Verification items for the finished model (mm, model axes). Coordinates: 2 decimals unless noted, no trailing zeros. Write each loop counter-clockwise with the first axis right and the second up, starting at its lowest first coordinate (ties: lowest second). Pieces come first, ordered by that corner, then holes. Notation, with made-up numbers: (70, -32.5) - (117, -32.5) arc R13 cw to (117, -17.5) - close; hole circle Ø3 at (-0.5, -23). An arc over 180 degrees is marked (long way). Answer as CSV lines item,"result". Start each with the question number.
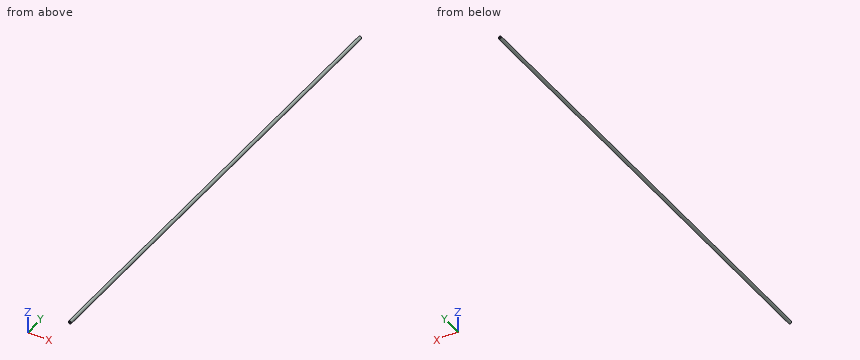
Autodesk Inventor part; units mm, degrees
ref_plane "YZ Plane" through (0, 0, 0) normal (1, 0, 0) x (0, 1, 0)
ref_plane "XZ Plane" through (0, 0, 0) normal (0, 1, 0) x (-1, 0, 0)
ref_plane "XY Plane" through (0, 0, 0) normal (0, 0, 1) x (1, 0, 0)
sketch "Sketch1" plane through (0, 0, 0) normal (0, 1, 0) x (-1, 0, 0)
  circle A0 centre (0, 0) radius 7
  circle A1 centre (0, 0) radius 3
  dimension "d0" = 14
  dimension "d1" = 6
extrude "Extrusion1" add sketch "Sketch1" along normal blind 1000 contours A0 | A1
extrude "Extrusion2" cut sketch "Sketch1" along normal blind 50 contours A1
chamfer "Chamfer1" distance 1 angle 45 1 edges at (7, 0, 0)
mirror "Mirror1" about plane through (0, 1000, 0) normal (0, 1, 0) of "Extrusion1", "Extrusion2", "Chamfer1"
properties part number "Tengely"
1. Cross-section at B-B (z = 0). Record the cut outline in (x, y), and give its area (3 significant figures).
2. Scan lines: line 1 along Z through (x, y) = (0, 38.5); line 2 along Z through (x, y) = (-1.75, 421); line 3 along X through (y, z) = (581, -1). Record each from-to range of solid material in increasing order. Write a range as from..to.
3. Depth check by flat-ended pin: P1, Ø5, axis at x = 0, z = 0, coming from the +Y side; P2, Ø1, axis at y = 1084.5, z = -4.5, coming from the -X side; P3, Ø3.5, axis at x = 0, z = 0, coming from the -Y side. Enter the tip coordinate at first touch or a pass-through.
4. Cross-section at C-C (y = 1081). Record the cut outline in (x, z).
5. Cross-section at A-A (x = 0). Record the cut outline in (y, z).
Completed:
1,outline,"(-7, 1) - (-6, 0) - (-3, 0) - (-3, 50) - (3, 50) - (3, 0) - (6, 0) - (7, 1) - (7, 1999) - (6, 2000) - (3, 2000) - (3, 1950) - (-3, 1950) - (-3, 2000) - (-6, 2000) - (-7, 1999) - close"
1,area,"27,400 mm2"
2,line 1,"z = -7..-3, 3..7"
2,line 2,"z = -6.78..6.78"
2,line 3,"x = -6.93..6.93"
3,P1,"stops at y = 1950"
3,P2,"stops at x = -5.74"
3,P3,"stops at y = 50"
4,outline,"circle Ø14 at (0, 0)"
5,outline,"(0, -6) - (1, -7) - (1999, -7) - (2000, -6) - (2000, -3) - (1950, -3) - (1950, 3) - (2000, 3) - (2000, 6) - (1999, 7) - (1, 7) - (0, 6) - (0, 3) - (50, 3) - (50, -3) - (0, -3) - close"
